```python
from build123d import *

# Parameters (mm, degrees)
SKETCH_3_W          = 186
SKETCH_3_H          = 8
EXTRUDE_1_DEPTH     = 119
SKETCH_9_R          = 2.5
CUT_EXTRUDE_1_DEPTH = 5
SKETCH_10_W         = 172
SKETCH_10_H         = 112
CUT_EXTRUDE_2_DEPTH = 3.5
SKETCH_11_W         = 120
SKETCH_11_H         = 60
CUT_EXTRUDE_3_DEPTH = 10
SKETCH_12_W         = 182
SKETCH_12_H         = 117
CUT_EXTRUDE_4_DEPTH = 2
SKETCH_15_W         = 25
SKETCH_15_H         = 2
CUT_EXTRUDE_8_DEPTH = 12
SKETCH_13_R         = 2.4
CUT_EXTRUDE_7_DEPTH = 12
MIRROR_START        = -14.334518618
MIRROR_3_DEPTH      = 20.078011551
FILLET_1_R          = 3


# Read off the part's stored shape, not the designer's step: 镜向3
with BuildPart() as part:
    # 草图1 → 放样1 section 0
    with BuildSketch(Plane(origin=(0, 0, 0), x_dir=(1, 0, 0), z_dir=(0, 1, 0))):
        with BuildLine():
            Line((-105, 20), (105, 20))
            Line((105, 20), (105, -20))
            Line((105, -20), (-105, -20))
            Line((-105, -20), (-105, 20))
        make_face()
    # 草图2 → 放样1 section 1
    with BuildSketch(Plane(origin=(0, 18, 0), x_dir=(1, 0, 0), z_dir=(0, 1, 0))):
        with BuildLine():
            Line((-95, 17.5), (95, 17.5))
            Line((95, 17.5), (95, -17.5))
            Line((95, -17.5), (-95, -17.5))
            Line((-95, -17.5), (-95, 17.5))
        make_face()
    loft()

    # 草图3 → 凸台-拉伸1 (add)
    with BuildSketch(Plane(origin=(0, 18, 0), x_dir=(1, 0, 0), z_dir=(0, 1, 0))):
        Rectangle(SKETCH_3_W, SKETCH_3_H)
    extrude(amount=EXTRUDE_1_DEPTH)

    # 草图5 → 切除-放样2 section 0
    with BuildSketch(Plane.XZ):
        with BuildLine():
            Line((-85, 15), (85, 15))
            Line((85, 15), (85, -15))
            Line((85, -15), (-85, -15))
            Line((-85, -15), (-85, 15))
        make_face()
    # 草图7 → 切除-放样2 section 1
    with BuildSketch(Plane(origin=(0, 11, 0), x_dir=(1, 0, 0), z_dir=(0, 1, 0))):
        with BuildLine():
            Line((-75, 12.5), (75, 12.5))
            Line((75, 12.5), (75, -12.5))
            Line((75, -12.5), (-75, -12.5))
            Line((-75, -12.5), (-75, 12.5))
        make_face()
    loft(mode=Mode.SUBTRACT)

    # 草图9 → 切除-拉伸1 (cut)
    with BuildSketch(Plane.XZ):
        with Locations(Location((95, 15, 0), (0, 0, 270))):
            Circle(SKETCH_9_R)
        with Locations(Location((-95, 15, 0), (0, 0, 270))):
            Circle(SKETCH_9_R)
        with Locations(Location((-95, -15, 0), (0, 0, 270))):
            Circle(SKETCH_9_R)
        with Locations(Location((95, -15, 0), (0, 0, 270))):
            Circle(SKETCH_9_R)
    extrude(amount=-CUT_EXTRUDE_1_DEPTH, mode=Mode.SUBTRACT)

    # 草图10 → 切除-拉伸2 (cut)
    with BuildSketch(Plane.XY.offset(4)):
        with Locations((0, 74)):
            Rectangle(SKETCH_10_W, SKETCH_10_H)
    cut_extrude_2 = extrude(amount=-CUT_EXTRUDE_2_DEPTH, mode=Mode.SUBTRACT)

    # 草图11 → 切除-拉伸3 (cut)
    with BuildSketch(Plane.XY.offset(0.5)):
        with Locations((0, 77.5)):
            Rectangle(SKETCH_11_W, SKETCH_11_H)
    extrude(amount=-CUT_EXTRUDE_3_DEPTH, mode=Mode.SUBTRACT)

    # 草图12 → 切除-拉伸4 (cut)
    with BuildSketch(Plane.XY.offset(4)):
        with Locations((0, 76.5)):
            Rectangle(SKETCH_12_W, SKETCH_12_H)
    cut_extrude_4 = extrude(amount=-CUT_EXTRUDE_4_DEPTH, mode=Mode.SUBTRACT)

    # 草图15 → 切除-拉伸8 (cut)
    with BuildSketch(Plane(origin=(0, 18, 0), x_dir=(1, 0, 0), z_dir=(0, 1, 0))):
        with Locations((0, -1.5)):
            Rectangle(SKETCH_15_W, SKETCH_15_H)
    cut_extrude_8 = extrude(amount=-CUT_EXTRUDE_8_DEPTH, mode=Mode.SUBTRACT)

    # 镜向1: 切除-拉伸2, 切除-拉伸4, 切除-拉伸8 across plane
    add(cut_extrude_2.mirror(Plane.XY), mode=Mode.SUBTRACT)
    add(cut_extrude_4.mirror(Plane.XY), mode=Mode.SUBTRACT)
    add(cut_extrude_8.mirror(Plane.XY), mode=Mode.SUBTRACT)

    # 草图13 → 切除-拉伸7 (cut)
    with BuildSketch(Plane.XY.offset(2)):
        with Locations((88.5, 131.5)):
            Circle(SKETCH_13_R)
        with Locations((88.5, 21.5)):
            Circle(SKETCH_13_R)
        with Locations((-88.5, 21.5)):
            Circle(SKETCH_13_R)
        with Locations((-88.5, 131.5)):
            Circle(SKETCH_13_R)
    extrude(amount=-CUT_EXTRUDE_7_DEPTH, mode=Mode.SUBTRACT)

    # 草图17 → 切除-放样3 section 0
    with BuildSketch(Plane(origin=(0, 18, 0), x_dir=(1, 0, 0), z_dir=(0, 1, 0))):
        with BuildLine():
            Line((87, 17.5), (95, 17.5))
            Line((95, 17.5), (95, 9.5))
            Line((95, 9.5), (87, 17.5))
        make_face()
    # 草图18 → 切除-放样3 section 1
    with BuildSketch(Plane(origin=(0, 0, 0), x_dir=(1, 0, 0), z_dir=(0, 1, 0))):
        with BuildLine():
            Line((103, 20), (105, 20))
            Line((105, 20), (105, 18))
            Line((105, 18), (103, 20))
        make_face()
    loft_3 = loft(mode=Mode.SUBTRACT)

    # 镜向2: 切除-放样3 across plane
    add(loft_3.mirror(Plane(origin=(0, 0, 0), x_dir=(0, 0, 1), z_dir=(1, 0, 0))), mode=Mode.SUBTRACT)

    # 镜向3 outline → 镜向3 (cut)
    with BuildSketch(Plane(origin=(0, 0, 0), x_dir=(1, 0, 0), z_dir=(0, 0.6973549598034537, -0.7167259309091051)).offset(MIRROR_START)):
        Polygon((-84.282271503, -27), (-87, -25.104778553), (-105, -12.552389276), (-106, -11.855034316), (-106, -27), align=None)
        Polygon((87, -25.104778553), (84.282271503, -27), (106, -27), (106, -11.855034316), (105, -12.552389276), align=None)
    extrude(amount=MIRROR_3_DEPTH, mode=Mode.SUBTRACT)

    # 圆角1
    fillet_1_edges = [part.edges().sort_by_distance(p)[0] for p in [
        (93, 137, 0),
        (-93, 137, 0),
    ]]
    fillet(fillet_1_edges, radius=FILLET_1_R)


solid = part.part
```
The listing builds one solid part. Answer for the finished solid, in the listing's coordinates (mm). A direction names the side the tool comes from. Coordinates: 2 decimals unless noted, no trailing zeros. Write each loop counter-clockwise with the first axis right and the second up, starting at its lowest first coordinate (ties: lowest second). Pieces come first, ordered by that corner, then holes. Notation, with made-up numbers: (-35.5, 41) - (13.5, 41) arc R28 ccw to (13.5, 74) - close; hole circle Ø7 at (7, 33). An arc over 180 degrees is marked (long way). Return JSON: item names as keys, results as strings. Group by question number.
Q1. Find the intervals of material crossed by line 1 along X through (y, z) = (131.5, -0.9); line 2 along X through (y, z) = (60, -3); line 3 along Y through (x, z) = (-17.5, -2.5), in increasing order. Write a range as [from, to].
Q2. For a pull along Z with two mould halves and no side action, classify faces 5 (the flat face through (96.042, 10.964, 15.689)), 6 (the cylindrical face through (-92.52, 2.46, -14.67)), 7 (the cylindrical face through (-87.21, 133.524, 0.028)) as +Z half, -Z half, draft (parallel to the pull), parting line (faces both ways), or undercut.
Q3. Flat-ended cylindrical pins translate along their axes: pin 1 Ø9 at (y, z) = (68.5, -0.5) entering from -X; pin 2 Ø1 at (x, z) = (-40, -3) entering from -Y; pin 3 Ø10 at (x, y) = (-9, 46) entering from +Z; pin 4 Ø6.5 at (x, z) = (95, 15) entering from -Y. Find the tip coordinate at first contact, or state that the pin passes through.
Q4. Which of the six approach directions +Z, -Z, +X, -X, +Y, -Y give full straight-line access (tool end or side, diameter ignored) to faces 1 (the flat face through (-3, 18, 7)), 2 (the flat face through (-93, 75, 0)), 3 (the flat face through (93, 75, 0)), 4 (the flat face through (-95, 5, 15))?
Q5. The part is cut by section B-B on y = 21.5. Write down the section's boundary in (x, z).
Q6. The part is cut by section A-A on y = 99.5. Write down the section's boundary in (x, z), and give its area (3 significant figures).
Evaluation:
{
 "1": {"line 1": "x = [-93, -90.9], [-86.1, 86.1], [90.9, 93]", "line 2": "x = [-93, -91], [91, 93]", "line 3": "y = [11, 18], [135, 137]"},
 "2": {"face 5": "+Z half", "face 6": "undercut", "face 7": "draft"},
 "3": {"pin 1": "stops at x = -93", "pin 2": "stops at y = 11", "pin 3": "stops at z = 0.5", "pin 4": "stops at y = 0"},
 "4": {"face 1": "none", "face 2": "+Z, -Z, -X, +Y", "face 3": "+Z, -Z, +X, +Y", "face 4": "-Y"},
 "5": {"outline": "(-93, -4) - (-91, -4) - (-91, -2) - (-90.9, -2) - (-90.9, 2) - (-91, 2) - (-91, 4) - (-93, 4) - close; (-86.1, -2) - (-86, -2) - (-86, -0.5) - (86, -0.5) - (86, -2) - (86.1, -2) - (86.1, 2) - (86, 2) - (86, 0.5) - (-86, 0.5) - (-86, 2) - (-86.1, 2) - close; (90.9, -2) - (91, -2) - (91, -4) - (93, -4) - (93, 4) - (91, 4) - (91, 2) - (90.9, 2) - close"},
 "6": {"outline": "(-93, -4) - (-91, -4) - (-91, -2) - (-86, -2) - (-86, -0.5) - (-60, -0.5) - (-60, 0.5) - (-86, 0.5) - (-86, 2) - (-91, 2) - (-91, 4) - (-93, 4) - close; (60, -0.5) - (86, -0.5) - (86, -2) - (91, -2) - (91, -4) - (93, -4) - (93, 4) - (91, 4) - (91, 2) - (86, 2) - (86, 0.5) - (60, 0.5) - close", "area": "124 mm2"}
}
